CAD build for the part. Positions are in the model's coordinates, mm. A direction names the side the tool comes from. Round coordinates to 2 decimals unless told otherwise and drop trailing zeros. Order: outer loops, then holes, each group sorted by start corner. A loop starts at its lowest first (then second) coordinate and runs counter-clockwise, first axis right, second up. Notation, with made-up numbers: (68, 26.5) -> (115, 26.5) arc R16 ccw to (115, 36.5) -> close; hole circle Ø11 at (10, 80). An arc over 180 degrees is marked (long way). Return JSON: item names as keys, results as strings. Group by question number.
Q1. Which spindle directions (+Z, -Z, +X, -X, +Y, -Y) get a long thin tool onto all of the face, cutting with end or side? Do faces 1 (the flat face through (129, 30, 13)), 2 (the cylindrical face through (1.282, 30.766, 13.978)), 3 (the cylindrical face through (46.33, -9.01, 42.22)). Say none if no direction does.
Q2. Mould opens along Z. For faces 4 (the flat face through (128.591, -27.465, 41.139)), 5 (the cylindrical face through (128.49, 25.343, 38.794)), 6 (the flat face through (-7, -33, 14)), 7 (the cylindrical face through (128.49, -21.657, 38.794)) say: +Z half, -Z half, draft (parallel to the pull), parting line (faces both ways), or undercut.
Q3. Flat gauge pins, fed straight in: pin 1 (15 mm diameter, centred on y = 16.5, z = 36, fed in from -X); pin 2 (8 mm diameter, centred on x = 27.5, y = 15.5, fed in from -Z); pin 3 (6 mm diameter, centred on y = -13.5, z = -6.5, fed in from +X); pin 4 (6 mm diameter, centred on x = 128.5, z = 12.5, fed in from -Y). Where does each tip first touch, or does it go through?
Q4. Probe line 1 along Z through (x, y) = (130, 23.5); line 2 along X through (y, z) = (-24, 34.5); line 3 along X through (y, z) = (15, 3.5). List the from-to ranges inside material, lowest first.
Q5. Cut at A-A (y = -23). Count the separate pieces of the cut face and the enclosed holes in it, then the cut area to 3 significant figures.
Q6. Cut at B-B (x = -21.5). Write the cut outline in (y, z), then the cut area to 3 significant figures.
from build123d import *

# Parameters (mm, degrees)
F2_W      = 60
F2_H      = 60
F3_DEPTH  = 7.25
F5_D      = 5
F6_SIZE   = 5
F7_R      = 5
F8_R      = 1
F10_R     = 8.5
F11_DEPTH = 33
F12_R     = 1


with BuildPart() as f1:
    # F0 (on Front) → F1 (revolve)
    with BuildSketch(Plane.XZ):
        Polygon((-35.0844461756, 13.6041676658), (157.1655538244, 13.6041676658), (157.1655538244, 18.6041676658), (132.1655538244, 18.6041676658), (132.1655538244, 43.6041676658), (-35.0844461756, 43.6041676658), align=None)
    revolve(axis=Axis((57.2006537472, 0, 13.6041676658), (1, 0, 0)))

    # F2 (on face) → F3 (join)
    with BuildSketch(Plane.YZ.offset(132.1655538244)):
        with Locations((0, 13.6041676658)):
            Rectangle(F2_W, F2_H)
    extrude(amount=-F3_DEPTH)

    # F5 (through all)
    with Locations(Plane.YZ.offset(132.1655538244)):
        with Locations((-23.5, 37.1041676658), (23.5, 37.1041676658), (-23.5, -9.8958323342), (23.5, -9.8958323342)):
            Hole(F5_D / 2)

    # F6
    f6_edges = [f1.edges().sort_by_distance(p)[0] for p in [
        (128.540554, 30, 43.604168),
        (128.540554, 30, -16.395832),
        (128.540554, -30, 43.604168),
        (128.540554, -30, -16.395832),
    ]]
    chamfer(f6_edges, length=F6_SIZE)

    # F7
    f7_edges = [f1.edges().sort_by_distance(p)[0] for p in [
        (-35.084446, 0, -16.395832),
    ]]
    fillet(f7_edges, radius=F7_R)

    # F8
    f8_edges = [f1.edges().sort_by_distance(p)[0] for p in [
        (157.165554, 0, 8.604168),
    ]]
    fillet(f8_edges, radius=F8_R)

    # F10 (on offset) → F11 (join, symmetric)
    with BuildSketch(Plane(origin=(0, 0, 0), x_dir=(-1, 0, 0), z_dir=(0, 1, 0))):
        with Locations((7.2094461756, 13.6041676658)):
            Circle(F10_R)
    extrude(amount=F11_DEPTH, both=True)

    # F12
    f12_edges = [f1.edges().sort_by_distance(p)[0] for p in [
        (1.290554, -33, 13.604168),
        (1.290554, 33, 13.604168),
    ]]
    fillet(f12_edges, radius=F12_R)


solid = f1.part
Solution:
{
 "1": {"face 1": "+Z, -Z, +X, +Y", "face 2": "+Y", "face 3": "none"},
 "2": {"face 4": "+Z half", "face 5": "undercut", "face 6": "draft", "face 7": "undercut"},
 "3": {"pin 1": "stops at x = -35.08", "pin 2": "stops at z = -14.1", "pin 3": "stops at x = 132.17", "pin 4": "stops at y = -30"},
 "4": {"line 1": "z = -16.4 to -12.4, -7.4 to 34.6, 39.6 to 43.6", "line 2": "x = 124.92 to 132.17", "line 3": "x = -35.08 to 132.17"},
 "5": {"separate pieces": "3", "enclosed holes": "0", "area": "6,510 mm²"},
 "6": {"outline": "circle Ø60 at (0, 13.6)", "area": "2,830 mm²"}
}
